Autodesk Inventor part; units mm, degrees
ref_plane "YZ Plane" through (0, 0, 0) normal (1, 0, 0) x (0, 1, 0)
ref_plane "XZ Plane" through (0, 0, 0) normal (0, 1, 0) x (-1, 0, 0)
ref_plane "XY Plane" through (0, 0, 0) normal (0, 0, 1) x (1, 0, 0)
sketch "Sketch1" plane through (0, 0, 0) normal (0, 1, 0) x (-1, 0, 0)
  circle A0 centre (0, 0) radius 10
  circle A1 centre (0, 0) radius 16
  dimension "d0" = 20
  dimension "d1" = 32
extrude "Extrusion1" add sketch "Sketch1" along normal blind 30
sketch "Sketch4" plane through (0, 0, 0) normal (0, 0, 1) x (1, 0, 0)
  circle A0 centre (0, 10) radius 3.45
  line L0 (-16, 0) -> (16, 0)
  point P0 (0, 0)
  dimension "d13" = 6.9
  dimension "d14" = 10
extrude "Extrusion4" cut sketch "Sketch4" along normal blind 30
sketch "Sketch5" plane through (0, 0, 0) normal (1, 0, 0) x (0, 1, 0)
  circle A0 centre (10, 0) radius 3.45
  line L0 (0, 16) -> (0, -16)
  point P0 (0, 0)
  dimension "d17" = 6.9
  dimension "d18" = 10
extrude "Extrusion5" cut sketch "Sketch5" against normal blind 30
sketch "Sketch6" plane through (0, 0, 0) normal (0, -1, 0) x (1, 0, 0)
  line L0 (-3.05, -9.5235) -> (3.05, -9.5235)
  line L1 (3.05, -9.5235) -> (3.05, -12.5735)
  line L2 (3.05, -12.5735) -> (-3.05, -12.5735)
  line L3 (-3.05, -12.5735) -> (-3.05, -9.5235)
  circle A0 centre (0, 0) radius 10
  dimension "d21" = 6.1
  dimension "d22" = 3.05
extrude "Extrusion6" cut sketch "Sketch6" against normal through all contours A0 L1 L2 L3 | L0 A0 picked at (0.3438, -9.6646)
sketch "Sketch9" plane through (0, 30, 0) normal (0, 1, 0) x (1, 0, 0)
  line L0 (-25, -25) -> (25, -25)
  line L1 (25, -25) -> (25, 25)
  line L2 (25, 25) -> (-25, 25)
  line L3 (-25, 25) -> (-25, -25)
  circle A0 centre (-17, -17) radius 3.265
  circle A1 centre (-17, 17) radius 3.265
  circle A2 centre (17, -17) radius 3.265
  circle A3 centre (17, 17) radius 3.265
  circle A4 centre (0, 0) radius 16
  dimension "d25" = 50
  dimension "d26" = 50
  dimension "d27" = 25
  dimension "d28" = 25
  dimension "d29" = 6.53
  dimension "d30" = 8
  dimension "d31" = 8
  dimension "d32" = 8
  dimension "d33" = 8
  dimension "d35" = 8
  dimension "d36" = 8
  dimension "d37" = 8
  dimension "d38" = 8
extrude "Extrusion7" add sketch "Sketch9" against normal blind 10
properties part number "1225a_Pinion Collar_V1" material "Aluminum 6061"
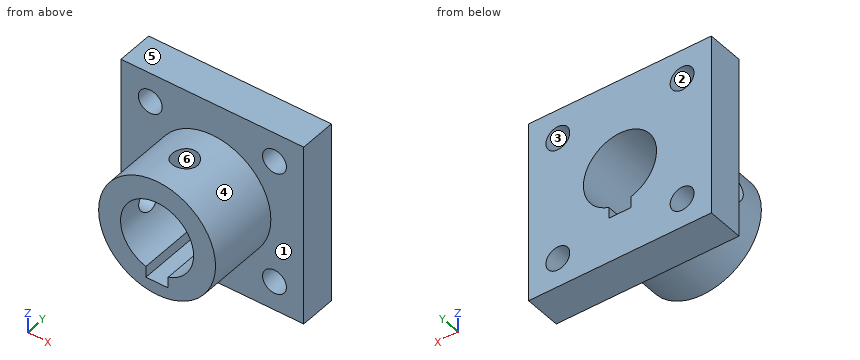
Verification items for the finished model (mm, model axes). Face numbers are marked on the shaded views. A direction names the side the tool comes from. Coordinates: 2 decimals unless noted, no trailing zeros. Write each loop counter-clockwise with the first axis right and the second up, starting at its lowest first coordinate (ties: lowest second). Pieces come first, ordered by that corner, then holes. Notation, with made-up numbers: (82, 42.5) - (104, 42.5) arc R24 ccw to (104, 63.5) - close; hole circle Ø5 at (44.5, 4). An arc over 180 degrees is marked (long way). Answer as a JSON object with one key per item and string values.
(1) Cross-section at B-B on y = 26.5. Give the number of separate pieces and of enclosed holes in the cut face, plus the area to 3 significant figures.
Report:
{"separate pieces": "1", "enclosed holes": "5", "area": "2,040 mm^2"}
(2) Gauge pin test, flat ends, axial feed: pin 1 Ø5 at (x, y) = (11, 12) entering from +Z; pin 2 Ø1.5 at (x, y) = (8.5, 3) entering from -Z; pin 3 Ø6 at (x, z) = (17, -17) entering from +Y; pin 4 Ø9 at (y, z) = (10, 0) entering from +X. Record the tip position at first contact, or that the pin passes through.
Report:
{"pin 1": "z = 13.56", "pin 2": "z = -14", "pin 3": "through", "pin 4": "x = 16"}
(3) Mould release check, pull along X, two halves, no side actions. Record for the marked faces 1, 2, 3 and 4: pulls with the +X half, pulls with the -X half, needs draft (parallel to the pull), parting line crosses it, or undercut.
Report:
{"face 1": "needs draft", "face 2": "undercut", "face 3": "undercut", "face 4": "parting line crosses it"}
(4) Tool access check on the marked faces 5 and 6. Record the directions out of +Z, -Z, +X, -X, +Y, -Y that give a thin tool (end or side, any length) a straight path to the whole face; none if there is none.
Report:
{"face 5": "+Z, +X, -X, +Y, -Y", "face 6": "+Z"}
(5) Cross-section at D-D on z = -7. Record the cut outline in (x, y), plus the area to 3 significant figures.
Report:
{"outline": "(-25, 20) - (-14.39, 20) - (-14.39, 0) - (-7.14, 0) - (-7.14, 30) - (-25, 30) - close; (7.14, 0) - (14.39, 0) - (14.39, 20) - (25, 20) - (25, 30) - (7.14, 30) - close", "area": "647 mm^2"}
(6) Cross-section at C-C on x = -17. Record the cut outline in (y, z) (3 decimals).
Report:
{"outline": "(20, -25) - (30, -25) - (30, -20.265) - (20, -20.265) - close; (20, -13.735) - (30, -13.735) - (30, 13.735) - (20, 13.735) - close; (20, 20.265) - (30, 20.265) - (30, 25) - (20, 25) - close"}
(7) Cross-section at A-A on z = 0. Record the cut outline in (x, y), plus the area to 3 significant figures.
Report:
{"outline": "(-25, 20) - (-16, 20) - (-16, 13.45) - (-10, 13.45) - (-10, 30) - (-25, 30) - close; (-16, 0) - (-10, 0) - (-10, 6.55) - (-16, 6.55) - close; (10, 0) - (16, 0) - (16, 20) - (25, 20) - (25, 30) - (10, 30) - close", "area": "499 mm^2"}
(8) Thickness scan on line 1 along X through (y, z) = (26, 17) (3 decimals); line 2 along Z through (x, y) = (0.5, 14). Record the ranges inside material, lowest first.
Report:
{"line 1": "-25 to -20.265, -13.735 to 13.735, 20.265 to 25", "line 2": "-15.99 to -12.57, 9.99 to 15.99"}
